The listing builds one solid part. Answer for the finished solid, in the listing's coordinates (mm). Give positions to 0.01 mm unless a question says otherwise; leave off trailing zeros. Order: outer loops, then holes, each group sorted by start corner. A loop starts at its lowest first (then second) coordinate and runs counter-clockwise, first axis right, second up. Notation, with made-up numbers: (32.5, 84) - (80.5, 84) arc R11 ccw to (80.5, 98) - close; hole circle Ø8 at (-13, -5.5). An arc over 180 degrees is marked (long way). Write each question's results on one line, items separated by ' | '. Start each with the question number.
1. Flat-ended cylindrical pins translate along their axes: pin 1 (4.5 mm diameter, centred on x = 30, z = 102, fed in from -Y); pin 2 (6.5 mm diameter, centred on x = 41, z = 68, fed in from +Y); pin 3 (1.5 mm diameter, centred on y = 1.5, z = -18, fed in from +X); pin 4 (0.9 mm diameter, centred on x = -80.5, y = 2, fed in from -Z). Find the tip coordinate at first contact, or state that the pin passes through.
2. Section B-B (z = -55) is taken. Give the vertices of the cut face in (x, y), and give its area (3 significant figures).
3. Find the intervals of material crossed by L1, parallel to Z at x = 70, y = 0.8; L2, parallel to X at y = 1.1, z = 68; L3, parallel to X at y = 1.05, z = -14, in increasing order.
4. Determine the mould class of faces 1 (the face through (1, 3, 2)), 2 (the face through (-29.67, 1.48, 99.52)) for opening direction X: released by +X, released by -X, zero draft, split by the parting line, or undercut.
5. Section A-A (y = 0.6) is taken. State how many separate pieces and enclosed holes the cut face has, and give its area (3 significant figures).
Autodesk Inventor part; units mm, degrees
ref_plane "YZ Plane" through (0, 0, 0) normal (1, 0, 0) x (0, 1, 0)
ref_plane "XZ Plane" through (0, 0, 0) normal (0, 1, 0) x (-1, 0, 0)
ref_plane "XY Plane" through (0, 0, 0) normal (0, 0, 1) x (1, 0, 0)
sketch "Sketch1" plane through (0, 0, 0) normal (0, 1, 0) x (-1, 0, 0)
  line L0 (75, 132) -> (-75, 132)
  line L1 (-75, -132) -> (75, -132)
  line L2 (75, 132) -> (-75, -132) construction
  line L3 (-75, 132) -> (75, -132) construction
  line L4 (75, 92) -> (85, 92)
  line L5 (85, 92) -> (85, 67)
  line L6 (85, 67) -> (75, 67)
  line L7 (75, 92) -> (75, 132)
  line L8 (0, 0) -> (94, 0)
  line L9 (75, -92) -> (85, -92)
  line L10 (85, -92) -> (85, -67)
  line L11 (85, -67) -> (75, -67)
  line L12 (75, -132) -> (75, -92)
  line L13 (75, -67) -> (75, 67)
  line L14 (-75, 92) -> (-85, 92)
  line L15 (-85, 92) -> (-85, 67)
  line L16 (-85, 67) -> (-75, 67)
  line L17 (-75, 132) -> (-75, 92)
  line L18 (-75, -92) -> (-85, -92)
  line L19 (-85, -92) -> (-85, -67)
  line L20 (-85, -67) -> (-75, -67)
  line L21 (-75, 67) -> (-75, -67)
  line L22 (-75, -92) -> (-75, -132)
  circle A0 centre (30, 102) radius 2.5
  circle A1 centre (-30, 102) radius 2.5
  dimension "d0" = 264
  dimension "d1" = 150
  dimension "d4" = 10
  dimension "d5" = 25
  dimension "d6" = 40
  dimension "d7" = 10
  dimension "d8" = 9
  dimension "d9" = 10
  dimension "d10" = 25
  dimension "d11" = 40
  dimension "d12" = 160
  dimension "d17" = 5
  dimension "d18" = 5
  dimension "d19" = 30
  dimension "d20" = 30
  dimension "d21" = 45
  dimension "d22" = 45
extrude "Extrusion1" add sketch "Sketch1" along normal blind 3
sketch "Sketch2" plane through (0, 3, 0) normal (0, 1, 0) x (1, 0, 0)
  line L0 (-86, -72) -> (86, -72)
  line L1 (-75, -132) -> (75, -132)
  line L2 (45, -72) -> (45, 18)
  line L3 (75, -67) -> (75, 67)
  line L4 (45, 18) -> (-44, 18)
  line L5 (-44, 18) -> (-44, -72)
  line L6 (-75, 67) -> (-75, -67)
  circle A0 centre (41, -68) radius 2
  circle A1 centre (41, 14) radius 2
  circle A2 centre (-40, 14) radius 2
  circle A3 centre (-40, -68) radius 2
  circle A4 centre (70, 129.734) radius 2
  line L7 (75, 132) -> (-75, 132)
  circle A5 centre (70, 37.266) radius 2
  circle A6 centre (-23.148, 129.734) radius 2
  circle A7 centre (-23.148, 37.266) radius 2
  point P0 (0, 0)
  dimension "d15" = 60
  dimension "d16" = 30
  dimension "d23" = 90
  dimension "d25" = 4
  dimension "d26" = 4
  dimension "d27" = 4
  dimension "d28" = 4
  dimension "d29" = 4
  dimension "d30" = 4
  dimension "d31" = 4
  dimension "d32" = 4
  dimension "d33" = 4
  dimension "d34" = 4
  dimension "d35" = 4
  dimension "d36" = 4
  dimension "d39" = 89
  dimension "d40" = 4
  dimension "d41" = 5
  dimension "d42" = 2.266
  dimension "d43" = 4
  dimension "d44" = 5
  dimension "d45" = 92.468
  dimension "d46" = 4
  dimension "d47" = 4
  dimension "d48" = 93.148
  dimension "d49" = 93.148
  dimension "d50" = 2.266
  dimension "d51" = 0
extrude "Extrusion2" cut sketch "Sketch2" against normal blind 3 contours A0 | A1 | A2 | A3 | A4 | A5 | A6 | A7
properties part number "bottom_part"
Reported:
1) pin 1: through | pin 2: y = 3 | pin 3: x = 75 | pin 4: z = -92
2) outline: (-75, 0) - (75, 0) - (75, 3) - (-75, 3) - close | area: 450 mm²
3) L1: -132 to -131.73, -127.73 to -39.27, -35.27 to 132 | L2: -85 to -42, -38 to 39, 43 to 85 | L3: -75 to -42, -38 to 39, 43 to 75
4) face 1: zero draft | face 2: undercut
5) separate pieces: 1 | enclosed holes: 10 | area: 40,500 mm²
